from build123d import *

# Parameters (mm, degrees)
BOSS_EXTRUDE1_DEPTH = 35
CUT_EXTRUDE1_DEPTH  = 70
SKETCH11_R          = 15
CUT_EXTRUDE2_DEPTH  = 20
SKETCH12_R          = 8
CUT_EXTRUDE3_DEPTH  = 30
CUT_EXTRUDE4_START  = -30
SKETCH13_R          = 8
CUT_EXTRUDE4_DEPTH  = 30


with BuildPart() as part:
    # Sketch1 → Boss-Extrude1 (new, symmetric)
    with BuildSketch(Plane.XY):
        Polygon((-46.019417476, 0), (-46.019417476, 40), (33.980582524, 40), (33.980582524, 0), (83.980582524, 0), (83.980582524, 15), (48.980582524, 15), (48.980582524, 55), (-61.019417476, 55), (-61.019417476, 15), (-96.019417476, 15), (-96.019417476, 0), align=None)
    extrude(amount=BOSS_EXTRUDE1_DEPTH, both=True)

    # Sketch2 → Cut-Extrude1 (cut)
    with BuildSketch(Plane(origin=(0, 15, 0), x_dir=(1, 0, 0), z_dir=(0, 1, 0))):
        with BuildLine():
            Line((65.087517656, 5), (83.980582524, 5))
            Line((83.980582524, 5), (83.980582524, -5))
            Line((83.980582524, -5), (65.087517656, -5))
            ThreePointArc((65.087517656, -5), (60.087517656, 0), (65.087517656, 5))
        make_face()
        with BuildLine():
            Line((-96.019417476, -5), (-96.019417476, 5))
            Line((-96.019417476, 5), (-77.126352608, 5))
            ThreePointArc((-77.126352608, 5), (-72.126352608, 0), (-77.126352608, -5))
            Line((-77.126352608, -5), (-96.019417476, -5))
        make_face()
    extrude(amount=-CUT_EXTRUDE1_DEPTH, mode=Mode.SUBTRACT)

    # Loft1: read off the stored shape, not the designer's step
    # Loft1: loft between two sections, ruled curve by curve
    loft1_from = [
        Edge.make_bspline([(-38.292502188, 105, 13.54429781), (-65.381097807, 105, -51.001871615), (-0.834928382, 105, -78.090467234), (26.253667237, 105, -13.54429781), (53.342262856, 105, 51.001871615), (-11.203906569, 105, 78.090467234), (-38.292502188, 105, 13.54429781)], [0, 0, 0, 0, 0.5, 0.5, 0.5, 1, 1, 1, 1], 3, [1, 0.333333333, 0.333333333, 1, 0.333333333, 0.333333333, 1]),
    ]
    loft1_to = [
        Edge.make_bspline([(-26.008227644, 55, -0.668930523), (-24.670366599, 55, -40.64655086), (15.307253739, 55, -39.308689814), (13.969392693, 55, 0.668930523), (12.631531647, 55, 40.64655086), (-27.34608869, 55, 39.308689814), (-26.008227644, 55, -0.668930523)], [0, 0, 0, 0, 0.5, 0.5, 0.5, 1, 1, 1, 1], 3, [1, 0.333333333, 0.333333333, 1, 0.333333333, 0.333333333, 1]),
    ]
    loft1 = Solid(Shell([*[Face.make_surface_from_curves(loft1_from[k], loft1_to[k]) for k in range(1)], Face(Wire(loft1_from)), Face(Wire(loft1_to))]))
    add(loft1)

    # Sketch11 → Cut-Extrude2 (cut)
    with BuildSketch(Plane(origin=(0, 105, 0), x_dir=(1, 0, 0), z_dir=(0, 1, 0))):
        with Locations(Location((-6.019417476, 0, 0), (0, 0, 270))):
            Circle(SKETCH11_R)
    extrude(amount=-CUT_EXTRUDE2_DEPTH, mode=Mode.SUBTRACT)

    # Sketch12 → Cut-Extrude3 (cut)
    with BuildSketch(Plane.XZ.offset(-40)):
        with Locations(Location((-6.019417476, 0, 0), (0, 0, 270))):
            Circle(SKETCH12_R)
    extrude(amount=-CUT_EXTRUDE3_DEPTH, mode=Mode.SUBTRACT)

    # Sketch13 → Cut-Extrude4 (cut)
    with BuildSketch(Plane(origin=(0, 85, 0), x_dir=(1, 0, 0), z_dir=(0, 1, 0)).offset(CUT_EXTRUDE4_START)):
        with Locations(Location((-6.019417476, 0, 0), (0, 0, 90))):
            Circle(SKETCH13_R)
    extrude(amount=CUT_EXTRUDE4_DEPTH, mode=Mode.SUBTRACT)


solid = part.part
Could you check a few things on this model? Use its own coordinates, in mm. A direction names the side the tool comes from. Give positions to 0.01 mm unless a question says otherwise; leave off trailing zeros. Order: outer loops, then holes, each group sorted by start corner. A loop starts at its lowest first (then second) coordinate and runs counter-clockwise, first axis right, second up. Notation, with made-up numbers: (12.5, 73) - (39.5, 73) arc R16 cw to (39.5, 90) - close; hole circle Ø11 at (73, 11). An arc over 180 degrees is marked (long way). Return JSON: item names as keys, results as strings. Group by question number.
Q1. Please list where these lines run through material, in increasing order: line 1 along Z through (x, y) = (75, 10); line 2 along X through (y, z) = (18, -7.5); line 3 along Y through (x, z) = (31, -26). Write a range as [from, to].
Q2. Thinking about a two-plate mould opening in X: for faces 1 (the face through (-10.887, 62.185, 6.349)), 2 (the face through (48.981, 35, 0)), 3 (the face through (-19, 105, -11)), which applies, pulls with the +X half, pulls with the -X half, needs draft (parallel to the pull), parting line crosses it, or undercut?
Q3. Which directions (+Z, -Z, +X, -X, +Y, -Y) give clear straight access to the entire face, cutting with the end or side of a thin tool? Please do faces 4 (the face through (74, 8, -5)), 5 (the face through (-70, 15, 0)), 6 (the face through (-15.15, 95.14, -11.9)), 7 (the face through (-86, 8, 5)), 8 (the face through (-6.6, 40, 8.3)).
Q4. Will these pins go through, and if not, where does the flat tip stop? pin 1 Ø12 at (y, z) = (27, 15.5) entering from +X; pin 2 Ø24 at (x, z) = (-11, 5.5) entering from +Y; pin 3 Ø6 at (x, z) = (-20, -0.5) entering from -Y; pin 4 Ø4 at (x, y) = (-9, 70) entering from -Z.
Q5. Suppose I cut it at A-A, the plane y = 49. Please give me the cut outline in (x, z), and give its area (3 significant figures).
Resolved:
{
 "1": {"line 1": "z = [-35, -5], [5, 35]", "line 2": "x = [-61.02, -46.02], [33.98, 48.98]", "line 3": "y = [40, 55]"},
 "2": {"face 1": "undercut", "face 2": "pulls with the +X half", "face 3": "needs draft"},
 "3": {"face 4": "+X, +Y, -Y", "face 5": "+Z, -Z, -X, +Y", "face 6": "+Y", "face 7": "-X, +Y, -Y", "face 8": "+Z, -Z, -Y"},
 "4": {"pin 1": "stops at x = 48.98", "pin 2": "stops at y = 105", "pin 3": "stops at y = 40", "pin 4": "stops at z = -24.38"},
 "5": {"outline": "(-61.02, -35) - (48.98, -35) - (48.98, 35) - (-61.02, 35) - close; hole circle Ø16 at (-6.02, 0)", "area": "7,500 mm2"}
}
